Source: three-view drawing plus pictorial views. Frame: mm from the lowest corner of the part. A direction names the side the tool comes from. Coordinates: 2 decimals unless noted, no trailing zeros. Write each loop counter-clockwise with the first axis right and the second up, starting at its lowest first coordinate (ties: lowest second). Pieces come first, ordered by that corner, then holes. Notation, with made-up numbers: M 69.25,-34.75 L 111.25,-34.75 A24 cw 111.25,-15.75 Z; hole C -19.75,83 d2. An arc over 180 degrees is marked long. Use CSV: the item, a comma, the result in double quotes.
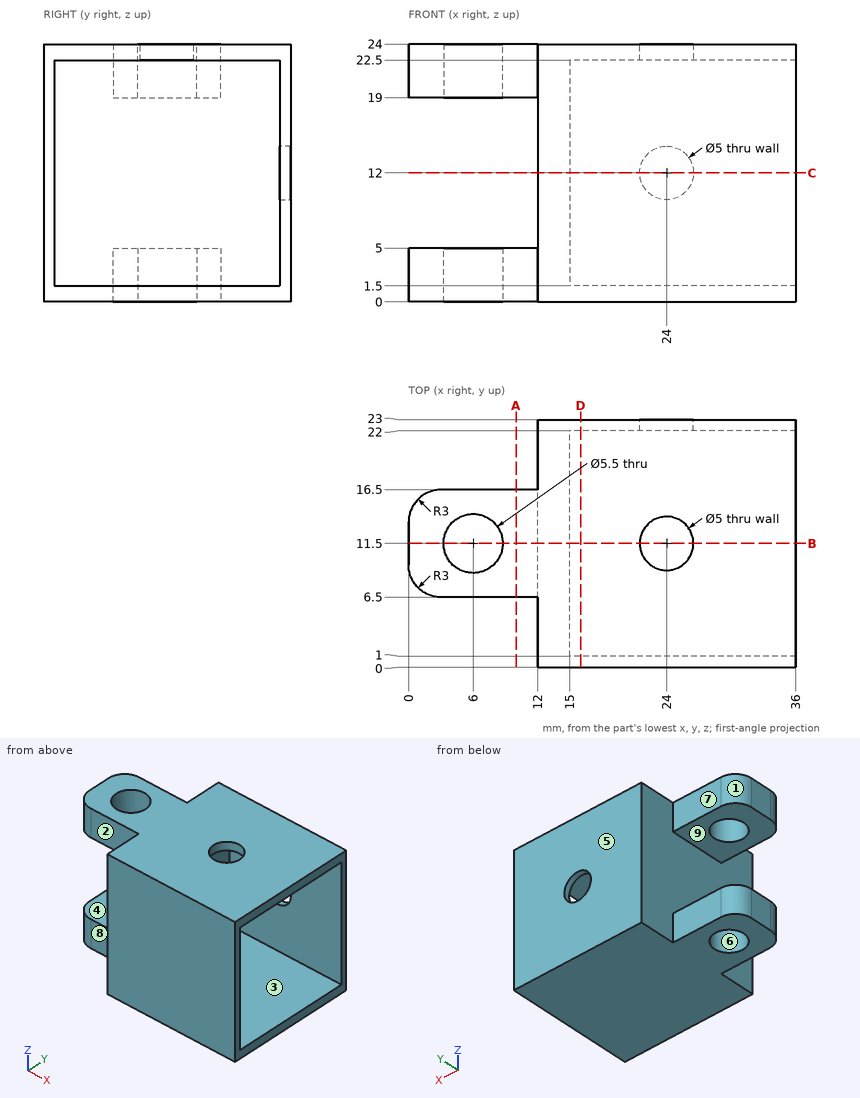
1. Section C-C (z = 12). Return loops of the section in (x, y).
Resolved:
outline,"M 12,0 L 36,0 L 36,1 L 15,1 L 15,22 L 21.5,22 L 21.5,23 L 12,23 Z; M 26.5,22 L 36,22 L 36,23 L 26.5,23 Z"
2. Section B-B (y = 11.5). Return loops of the section in (x, z), then the cut area to 4 significant figures.
Resolved:
outline,"M 0,0 L 3.25,0 L 3.25,5 L 0,5 Z; M 0,19 L 3.25,19 L 3.25,24 L 0,24 Z; M 8.75,0 L 36,0 L 36,1.5 L 15,1.5 L 15,22.5 L 21.5,22.5 L 21.5,24 L 8.75,24 L 8.75,19 L 12,19 L 12,5 L 8.75,5 Z; M 26.5,22.5 L 36,22.5 L 36,24 L 26.5,24 Z"
area,"192.5 mm^2"
3. Contact query for flat-ended pins moving along their axis: pin 1 Ø5 at (x, y) = (6, 11.5) entering from -Z; pin 2 Ø2 at (y, z) = (19.5, 12.5) entering from -X; pin 3 Ø4 at (x, z) = (9, 2.5) entering from -Y; pin 4 Ø1.5 at (x, z) = (6, 1.5) entering from +Y. Output: stop coordinate, or through.
Resolved:
pin 1,"passes through"
pin 2,"stops at x = 12"
pin 3,"stops at y = 6.5"
pin 4,"stops at y = 16.5"
4. Mould query, pull axis Y, two halves, no side actions, for the marked faces 1, 2, 3 and 4. Classes: pulls with the +Y half, pulls with the -Y half, needs draft (parallel to the pull), parting line crosses it, or undercut.
Resolved:
face 1,"pulls with the +Y half"
face 2,"pulls with the -Y half"
face 3,"undercut"
face 4,"needs draft"
5. Section D-D (x = 16). Return loops of the section in (y, z).
Resolved:
outline,"M 0,0 L 23,0 L 23,24 L 0,24 Z; hole M 1,1.5 L 22,1.5 L 22,22.5 L 1,22.5 Z"
6. Material intervals for line 1 (Z direction, x = 33.5, y = 2.75); line 2 (Y direction, x = 6, z = 2.3); line 3 (Y direction, x = 24, z = 22.8), sorted ascending. Write a range as [from, to].
Resolved:
line 1,"z = [0, 1.5], [22.5, 24]"
line 2,"y = [6.5, 8.75], [14.25, 16.5]"
line 3,"y = [0, 9], [14, 23]"
7. Access query for the marked faces 5, 6, 7, 8 and 9. Directions: +Z, -Z, +X, -X, +Y, -Y. A direction counts if a zero-diameter tool reaches every point of the face in a straight line with its end or side. Return the directions, or none.
Resolved:
face 5,"+Z, -Z, +X, -X, +Y"
face 6,"+Z, -Z"
face 7,"+Z, -Z, -X, +Y"
face 8,"+Z, -Z, -X, -Y"
face 9,"-X, +Y, -Y"
8. Section A-A (x = 10). Return loops of the section in (y, z), then the cut area to 3 significant figures.
Resolved:
outline,"M 6.5,0 L 16.5,0 L 16.5,5 L 6.5,5 Z; M 6.5,19 L 16.5,19 L 16.5,24 L 6.5,24 Z"
area,"100 mm^2"
